Input: part model. Units: mm. Frame: model coordinates. Face numbers are marked on the shaded views. A direction names the side the tool comes from. Give positions to 0.01 mm unless a question says otherwise; leave off trailing zeros. Write each loop counter-clockwise with the first axis right and the second up, starting at its lowest first coordinate (ties: lowest second). Pieces come first, ordered by that corner, then holes. Notation, with made-up numbers: (69, -11.5) -> (107, -11.5) arc R23 ccw to (107, -1.5) -> close; hole circle Ø1 at (50, 50.25). An arc over 180 degrees is marked (long way). Answer as a JSON object with one key per item and string values. Group by question number.
from build123d import *

# Parameters (mm, degrees)
SKETCH_1_R          = 2.5
EXTRUDE_1_DEPTH     = 4
SKETCH_2_W          = 4
SKETCH_2_H          = 50
EXTRUDE_2_DEPTH     = 20.7
SKETCH_3_R          = 2
CUT_EXTRUDE_1_DEPTH = 6.7
CUT_EXTRUDE_2_DEPTH = 10


with BuildPart() as part:
    # Эскиз1 → Бобышка-Вытянуть1 (new body)
    with BuildSketch(Plane.XY):
        Polygon((0, 0), (108, 0), (108, 50), (55, 50), (55, 68), (0, 68), align=None)
        with Locations((21, 57)):
            Circle(SKETCH_1_R, mode=Mode.SUBTRACT)
        with Locations((49, 57)):
            Circle(SKETCH_1_R, mode=Mode.SUBTRACT)
        with Locations((21, 11)):
            Circle(SKETCH_1_R, mode=Mode.SUBTRACT)
        with Locations((49, 11)):
            Circle(SKETCH_1_R, mode=Mode.SUBTRACT)
        with Locations((93, 25)):
            Circle(SKETCH_1_R, mode=Mode.SUBTRACT)
    extrude(amount=EXTRUDE_1_DEPTH)

    # Эскиз2 → Бобышка-Вытянуть2 (add)
    with BuildSketch(Plane.XY.offset(4)):
        with Locations((106, 25)):
            Rectangle(SKETCH_2_W, SKETCH_2_H)
    extrude(amount=-EXTRUDE_2_DEPTH)

    # Эскиз3 → Вырез-Вытянуть1 (cut)
    with BuildSketch(Plane(origin=(108, 0, 0), x_dir=(0, 0, -1), z_dir=(1, 0, 0))):
        with Locations((8.7, 45)):
            Circle(SKETCH_3_R)
        with Locations((8.7, 17)):
            Circle(SKETCH_3_R)
    extrude(amount=-CUT_EXTRUDE_1_DEPTH, mode=Mode.SUBTRACT)

    # Эскиз4 → Вырез-Вытянуть2 (cut)
    with BuildSketch(Plane(origin=(0, 0, 0), x_dir=(-1, 0, 0), z_dir=(0, 0, -1))):
        Polygon((0, 68), (-15, 68), (-15, 48), (-15, 28), (-10, 28), (-10, 58), (0, 58), align=None)
    extrude(amount=-CUT_EXTRUDE_2_DEPTH, mode=Mode.SUBTRACT)


solid = part.part
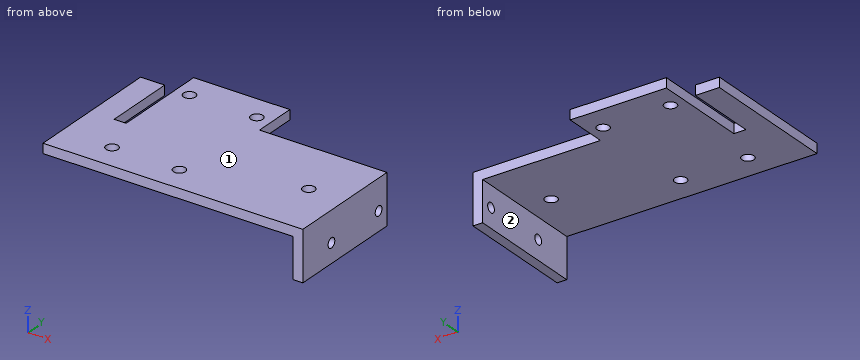
1. Section C-C (y = 33). Return the cut outline in (x, z).
2. Contact query for flat-ended pins moving along their axis: pin 1 Ø1.5 at (y, z) = (33.5, -5.5) entering from -X; pin 2 Ø1.2 at (x, z) = (2.5, 1) entering from +Y; pin 3 Ø2 at (x, z) = (13.5, 1.5) entering from +Y. Output: stop coordinate, or through.
3. Section D-D (z = 2.75). Return the cut outline in (x, y).
4. Section A-A (y = 11). Return the cut outline in (x, z).
5. Section B-B (x = 21). Return the cut outline in (y, z).
6. Reachability of the marked faces 1 and 2 from +Z, -Z, +X, -X, +Y, -Y: full face, straight path, thin tool, end or side. Return the list, or none.
7. Line query: line 1 (Y direction, x = 105.65, z = -8.7); line 2 (Y direction, x = 49, z = 0.85); line 3 (X direction, y = 30.5, z = 2.75). Output: solid intervals per line, ascending.
Working result:
{
 "1": {"outline": "(0, 0) -> (10, 0) -> (10, 4) -> (0, 4) -> close; (15, 0) -> (104, 0) -> (104, -16.7) -> (108, -16.7) -> (108, 4) -> (15, 4) -> close"},
 "2": {"pin 1": "stops at x = 104", "pin 2": "stops at y = 58", "pin 3": "stops at y = 28"},
 "3": {"outline": "(0, 0) -> (108, 0) -> (108, 50) -> (55, 50) -> (55, 68) -> (15, 68) -> (15, 28) -> (10, 28) -> (10, 58) -> (0, 58) -> close; hole circle Ø5 at (21, 11); hole circle Ø5 at (21, 57); hole circle Ø5 at (49, 11); hole circle Ø5 at (49, 57); hole circle Ø5 at (93, 25)"},
 "4": {"outline": "(0, 0) -> (18.5, 0) -> (18.5, 4) -> (0, 4) -> close; (23.5, 0) -> (46.5, 0) -> (46.5, 4) -> (23.5, 4) -> close; (51.5, 0) -> (104, 0) -> (104, -16.7) -> (108, -16.7) -> (108, 4) -> (51.5, 4) -> close"},
 "5": {"outline": "(0, 0) -> (8.5, 0) -> (8.5, 4) -> (0, 4) -> close; (13.5, 0) -> (54.5, 0) -> (54.5, 4) -> (13.5, 4) -> close; (59.5, 0) -> (68, 0) -> (68, 4) -> (59.5, 4) -> close"},
 "6": {"face 1": "+Z, +X, -X, +Y, -Y", "face 2": "-Z, -X, +Y, -Y"},
 "7": {"line 1": "y = 0 to 15, 19 to 43, 47 to 50", "line 2": "y = 0 to 8.5, 13.5 to 54.5, 59.5 to 68", "line 3": "x = 0 to 10, 15 to 108"}
}
